from build123d import *
from build123d.topology import SkipClean

# Parameters (mm, degrees)
SKETCH1_W           = 75
SKETCH1_H           = 75
SKETCH1_R           = 1.6
SKETCH1_R_2         = 3.1
BOSS_EXTRUDE1_DEPTH = 4
BOSS_EXTRUDE2_START = 4
SKETCH3_W           = 75
SKETCH3_H           = 75
SKETCH3_R           = 3.1
SKETCH3_R_2         = 1.6
BOSS_EXTRUDE2_DEPTH = 4
SKETCH5_R           = 5.05
SKETCH5_R_2         = 2.95
CUT_EXTRUDE1_DEPTH  = 6.1
FILLET2_R           = 5


with BuildPart() as part:
    # Sketch1 → Boss-Extrude1 (new body)
    with BuildSketch(Plane(origin=(0, 0, 0), x_dir=(1, 0, 0), z_dir=(0, 1, 0))):
        Rectangle(SKETCH1_W, SKETCH1_H)
        with Locations(Location((-32.5, 0, 0), (0, 0, 270))):
            Circle(SKETCH1_R, mode=Mode.SUBTRACT)
        with Locations(Location((-25.5, 0, 0), (0, 0, 90))):
            Circle(SKETCH1_R, mode=Mode.SUBTRACT)
        with Locations(Location((25.5, 0, 0), (0, 0, 270))):
            Circle(SKETCH1_R, mode=Mode.SUBTRACT)
        with Locations(Location((32.5, 0, 0), (0, 0, 90))):
            Circle(SKETCH1_R, mode=Mode.SUBTRACT)
        with Locations(Location((-7.5, -25.5, 0), (0, 0, 270))):
            Circle(SKETCH1_R_2, mode=Mode.SUBTRACT)
        with Locations(Location((7.5, -25.5, 0), (0, 0, 90))):
            Circle(SKETCH1_R_2, mode=Mode.SUBTRACT)
        with Locations(Location((7.5, 25.5, 0), (0, 0, 270))):
            Circle(SKETCH1_R_2, mode=Mode.SUBTRACT)
        with Locations(Location((-7.5, 25.5, 0), (0, 0, 90))):
            Circle(SKETCH1_R_2, mode=Mode.SUBTRACT)
    extrude(amount=BOSS_EXTRUDE1_DEPTH)

    # Sketch3 → Boss-Extrude2 (add)
    with SkipClean():  # the faces are left unmerged after this step: merging them gives an invalid solid
        with BuildSketch(Plane.XZ.offset(BOSS_EXTRUDE2_START)):
            Rectangle(SKETCH3_W, SKETCH3_H)
            with Locations(Location((-7.5, -25.5, 0), (0, 0, 270))):
                Circle(SKETCH3_R, mode=Mode.SUBTRACT)
            with Locations(Location((7.5, -25.5, 0), (0, 0, 270))):
                Circle(SKETCH3_R, mode=Mode.SUBTRACT)
            with Locations(Location((32.5, 0, 0), (0, 0, 270))):
                Circle(SKETCH3_R_2, mode=Mode.SUBTRACT)
            with Locations(Location((25.5, 0, 0), (0, 0, 270))):
                Circle(SKETCH3_R_2, mode=Mode.SUBTRACT)
            with Locations(Location((7.5, 25.5, 0), (0, 0, 270))):
                Circle(SKETCH3_R, mode=Mode.SUBTRACT)
            with Locations(Location((-7.5, 25.5, 0), (0, 0, 270))):
                Circle(SKETCH3_R, mode=Mode.SUBTRACT)
            with Locations(Location((-25.5, 0, 0), (0, 0, 270))):
                Circle(SKETCH3_R_2, mode=Mode.SUBTRACT)
            with Locations(Location((-32.5, 0, 0), (0, 0, 270))):
                Circle(SKETCH3_R_2, mode=Mode.SUBTRACT)
        extrude(amount=-BOSS_EXTRUDE2_DEPTH)

    # Sketch5 → Cut-Extrude1 (cut)
    with BuildSketch(Plane.XZ.offset(4)):
        with Locations(Location((-7.5, -25.5, 0), (0, 0, 270))):
            Circle(SKETCH5_R)
        with Locations(Location((7.5, -25.5, 0), (0, 0, 90))):
            Circle(SKETCH5_R)
        with Locations(Location((7.5, 25.5, 0), (0, 0, 270))):
            Circle(SKETCH5_R)
        with Locations(Location((-7.5, 25.5, 0), (0, 0, 90))):
            Circle(SKETCH5_R)
        with Locations(Location((-32.5, 0, 0), (0, 0, 270))):
            Circle(SKETCH5_R_2)
        with Locations(Location((-25.5, 0, 0), (0, 0, 270))):
            Circle(SKETCH5_R_2)
        with Locations(Location((25.5, 0, 0), (0, 0, 90))):
            Circle(SKETCH5_R_2)
        with Locations(Location((32.5, 0, 0), (0, 0, 90))):
            Circle(SKETCH5_R_2)
    extrude(amount=-CUT_EXTRUDE1_DEPTH, mode=Mode.SUBTRACT)

    # Fillet2
    fillet2_edges = [part.edges().sort_by_distance(p)[0] for p in [
        (-37.5, 0, -37.5),
        (37.5, 0, -37.5),
        (37.5, 0, 37.5),
        (-37.5, 0, 37.5),
    ]]
    fillet(fillet2_edges, radius=FILLET2_R)


solid = part.part
CAD build for the part. Positions are in the model's coordinates, mm. A direction names the side the tool comes from. Coordinates: 2 decimals unless noted, no trailing zeros. Order: outer loops, then holes, each group sorted by start corner. A loop starts at its lowest first (then second) coordinate and runs counter-clockwise, first axis right, second up.
Item 1: Drill centre lines: L1, parallel to X at y = 3.55, z = -25.5; L2, parallel to X at y = -0.25, z = -25.5; L3, parallel to Z at x = -11, y = 0.5. Where is each one in solid material? Low to high.
Check sheet entries:
L1: x = -37.5 to -10.6, -4.4 to 4.4, 10.6 to 37.5
L2: x = -37.5 to -12.55, -2.45 to 2.45, 12.55 to 37.5
L3: z = -37.5 to -29.14, -21.86 to 21.86, 29.14 to 37.5
Item 2: Two-plate mould, pull along Z, no slides. Class faces 1 (the face through (-36.07, -0.06, -36)), 2 (the face through (7.278, -0.993, -30.545)), 3 (the face through (-37.5, 0, 0)), 4 (the face through (-36.07, 0.06, 36)): +Z half, -Z half, draft (parallel to the pull), parting line (faces both ways), or undercut.
Check sheet entries:
face 1: -Z half
face 2: undercut
face 3: draft
face 4: +Z half
Item 3: Band-saw the part on A-A on z = -25.5. List the corners of the cut face in (x, y), plus the area to 3 significant figures.
Check sheet entries:
outline: (-37.5, -4) - (-12.55, -4) - (-12.55, 2.1) - (-10.6, 2.1) - (-10.6, 4) - (-37.5, 4) - close; (-4.4, 2.1) - (-2.45, 2.1) - (-2.45, -4) - (2.45, -4) - (2.45, 2.1) - (4.4, 2.1) - (4.4, 4) - (-4.4, 4) - close; (10.6, 2.1) - (12.55, 2.1) - (12.55, -4) - (37.5, -4) - (37.5, 4) - (10.6, 4) - close
area: 453 mm2
Item 4: 3-axis set-ups, long thin cutter, end or side, ignore diameter. For faces 5 (the face through (7.722, -0.993, 30.545)), 6 (the face through (-1, -4, 1)): which of +Z, -Z, +X, -X, +Y, -Y reach the whole face in a straight line?
Check sheet entries:
face 5: -Y
face 6: +Z, -Z, +X, -X, -Y
Item 5: Band-saw the part on C-C on x = -7.5. List the corners of the cut face in (y, z), plus the area to 3 significant figures.
Check sheet entries:
outline: (-4, -37.5) - (4, -37.5) - (4, -28.6) - (2.1, -28.6) - (2.1, -30.55) - (-4, -30.55) - close; (-4, -20.45) - (2.1, -20.45) - (2.1, -22.4) - (4, -22.4) - (4, 22.4) - (2.1, 22.4) - (2.1, 20.45) - (-4, 20.45) - close; (-4, 30.55) - (2.1, 30.55) - (2.1, 28.6) - (4, 28.6) - (4, 37.5) - (-4, 37.5) - close
area: 453 mm2
Item 6: Band-saw the part on D-D on x = 25.5. List the corners of the cut face in (y, z), plus the area to 3 significant figures.
Check sheet entries:
outline: (-4, -37.5) - (4, -37.5) - (4, -1.6) - (2.1, -1.6) - (2.1, -2.95) - (-4, -2.95) - close; (-4, 2.95) - (2.1, 2.95) - (2.1, 1.6) - (4, 1.6) - (4, 37.5) - (-4, 37.5) - close
area: 558 mm2
Item 7: Pin check, flat tips, straight feed: pin 1 Ø10 at (x, z) = (-7.5, -25.5) entering from +Y; pin 2 Ø6 at (x, z) = (-7.5, 25.5) entering from -Y; pin 3 Ø4 at (x, z) = (-25.5, 0) entering from -Y. Stop position of each tip, or through.
Check sheet entries:
pin 1: stops at y = 4
pin 2: passes through
pin 3: stops at y = 2.1
Item 8: Band-saw the part on B-B on y = -0.25. Give the number of separate pieces and of enclosed holes in the cut face, plus the area to 3 significant figures.
Check sheet entries:
separate pieces: 1
enclosed holes: 8
area: 5,170 mm2
